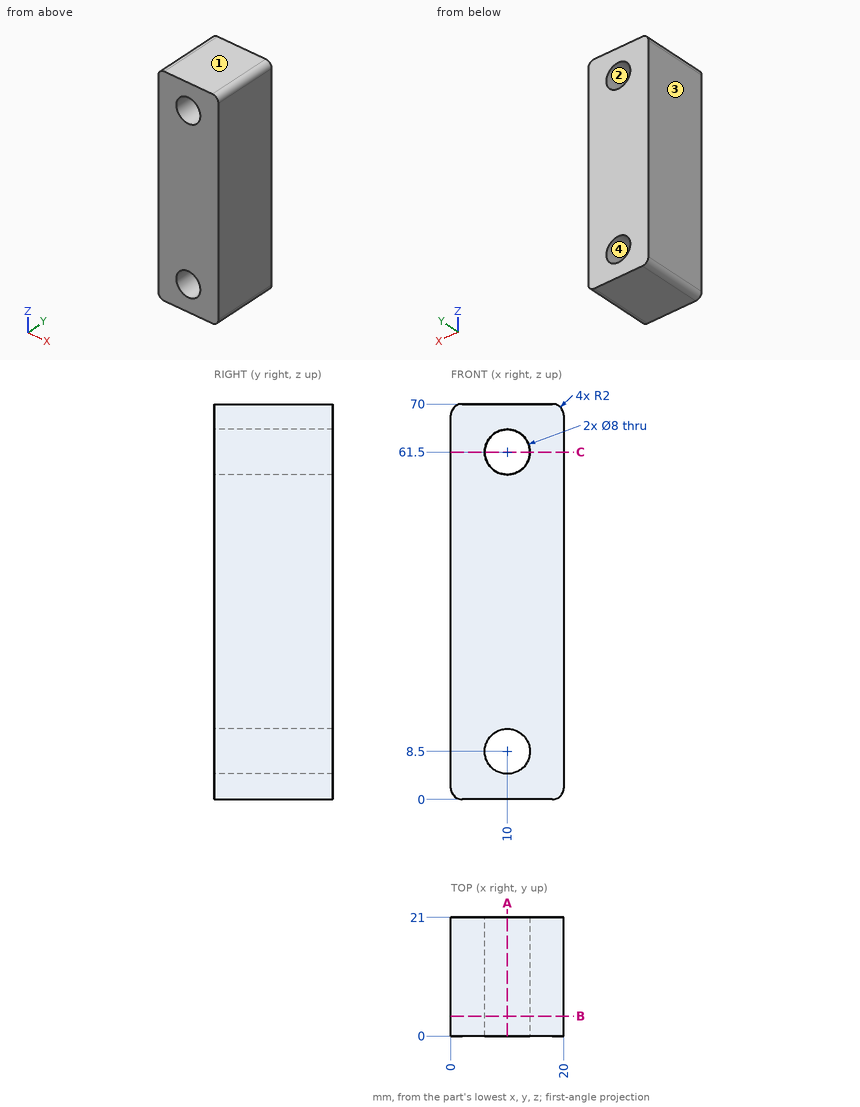
Check sheet for the drawn part. Datum: minimum x, y, z corner. Units: mm. Round coordinates to 2 decimals unless told otherwise and drop trailing zeros. Write each loop counter-clockwise with the first axis right and the second up, starting at its lowest first coordinate (ties: lowest second). Pieces come first, ordered by that corner, then holes. Notation, with made-up numbers: (-34, 67.25) - (-8, 67.25) arc R30 cw to (-8, 102.25) - close; hole circle Ø4 at (11, -17.75). An arc over 180 degrees is marked (long way). Return JSON: item names as keys, results as strings.
Q1. Cross-section at B-B (y = 3.5). Record the boundary of the cut face in (x, z).
Returned:
{"outline": "(0, 2) arc R2 ccw to (2, 0) - (18, 0) arc R2 ccw to (20, 2) - (20, 68) arc R2 ccw to (18, 70) - (2, 70) arc R2 ccw to (0, 68) - close; hole circle Ø8 at (10, 8.5); hole circle Ø8 at (10, 61.5)"}
Q2. Scan lines: L1, parallel to Z at x = 10, y = 13; L2, parallel to X at y = 17.25, z = 62; L3, parallel to Z at x = 18.25, y = 14.75. Record each from-to range of solid material in increasing order. Write a range as from..to.
Returned:
{"L1": "z = 0..4.5, 12.5..57.5, 65.5..70", "L2": "x = 0..6.03, 13.97..20", "L3": "z = 0.02..69.98"}
Q3. Draft check along Z on the marked faces 1, 2, 3 and 4. Enter one of: released by +Z, released by -Z, zero draft, split by the parting line, or undercut.
Returned:
{"face 1": "released by +Z", "face 2": "undercut", "face 3": "zero draft", "face 4": "undercut"}
Q4. Cross-section at C-C (z = 61.5). Record the boundary of the cut face in (x, y).
Returned:
{"outline": "(0, 0) - (6, 0) - (6, 21) - (0, 21) - close; (14, 0) - (20, 0) - (20, 21) - (14, 21) - close"}
Q5. Cross-section at A-A (x = 10). Record the boundary of the cut face in (y, z).
Returned:
{"outline": "(0, 0) - (21, 0) - (21, 4.5) - (0, 4.5) - close; (0, 12.5) - (21, 12.5) - (21, 57.5) - (0, 57.5) - close; (0, 65.5) - (21, 65.5) - (21, 70) - (0, 70) - close"}
Q6. Depth check by flat-ended pin: P1, Ø5, axis at x = 10, z = 61.5, coming from the -Y side. Enter the tip coordinate at first touch or a pass-through.
Returned:
{"P1": "passes through"}
